For this review, use the dimensioned drawing (mm, ordinates from the lowest corner) and the shaded views. A direction names the side the tool comes from. Give positions to 0.01 mm unless a question says otherwise; leave off trailing zeros. Order: outer loops, then holes, each group sorted by start corner. A loop starts at its lowest first (then second) coordinate and runs counter-clockwise, first axis right, second up. Notation, with made-up numbers: (-28, 67.25) -> (3, 67.25) arc R5 ccw to (3, 71.25) -> close; hole circle Ø2 at (89, 2). An arc over 180 degrees is marked (long way). Return JSON: item names as keys, results as strings.
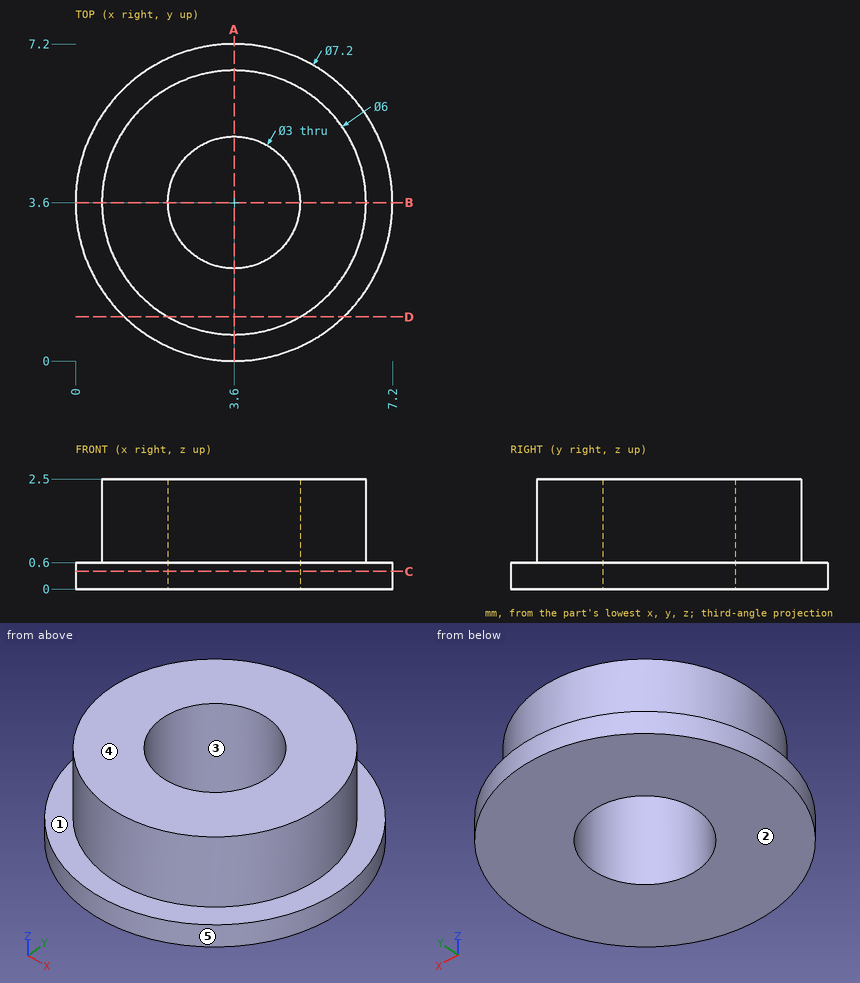
Item 1: Machinability: for the marked faces 1 and 2, which of the approach directions +Z, -Z, +X, -X, +Y, -Y give a long, thin tool a straight path to every point of the face, cutting with its end or side? Answer none if there is none.
Result set:
{"face 1": "+Z", "face 2": "-Z, +X, -X, +Y, -Y"}
Item 2: Wall thickness on L1, parallel to Y at x = 3.6, z = 1.2; L2, parallel to Y at x = 2.5, z = 2.15; L3, parallel to Z at x = 5.75, y = 6: over which ranges is each line inside the solid? List them lowest first. Write a range as [from, to].
Result set:
{"L1": "y = [0.6, 2.1], [5.1, 6.6]", "L2": "y = [0.81, 2.58], [4.62, 6.39]", "L3": "z = [0, 0.6]"}
Item 3: For pin 1 (1 mm diameter, centred on y = 2.5, z = 2, fed in from +X); pin 2 (1 mm diameter, centred on x = 3.5, z = 1, fed in from -Y); pin 3 (1.5 mm diameter, centred on y = 2.5, z = 0.5, fed in from +X); pin 4 (1 mm diameter, centred on y = 4, z = 1.5, fed in from -X), all flat-tipped, find the tip position at first contact; note any pin that passes through.
Result set:
{"pin 1": "stops at x = 6.54", "pin 2": "stops at y = 0", "pin 3": "stops at x = 7.18", "pin 4": "stops at x = 0.6"}
Item 4: Add section A-A (x = 3.6). Give the boundary of the cut face in (y, z), plus the area to 3 significant figures.
Result set:
{"outline": "(0, 0) -> (2.1, 0) -> (2.1, 2.5) -> (0.6, 2.5) -> (0.6, 0.6) -> (0, 0.6) -> close; (5.1, 0) -> (7.2, 0) -> (7.2, 0.6) -> (6.6, 0.6) -> (6.6, 2.5) -> (5.1, 2.5) -> close", "area": "8.22 mm^2"}
Item 5: Add section D-D (y = 1). Give the boundary of the cut face in (x, z), plus the area to 3 significant figures.
Result set:
{"outline": "(1.11, 0) -> (6.09, 0) -> (6.09, 0.6) -> (5.1, 0.6) -> (5.1, 2.5) -> (2.1, 2.5) -> (2.1, 0.6) -> (1.11, 0.6) -> close", "area": "8.68 mm^2"}
Item 6: Mouldability with a two-part tool opening along X and no side actions: class the marked faces 3, 4 and 5 as released by +X, released by -X, zero draft, split by the parting line, or undercut.
Result set:
{"face 3": "undercut", "face 4": "zero draft", "face 5": "split by the parting line"}
Item 7: Add section C-C (z = 0.4). Give the boundary of the cut face in (x, y).
Result set:
{"outline": "circle Ø7.2 at (3.6, 3.6); hole circle Ø3 at (3.6, 3.6)"}
